Geometry: see drawing. Coordinates: mm, zero at the bounding-box minimum. Give positions to 0.01 mm unless a question says otherwise; leave off trailing zeros. Write each loop counter-clockwise with the first axis right and the second up, starting at its lowest first coordinate (ties: lowest second). Pieces come first, ordered by that corner, then holes. Notation, with made-up numbers: (11, 64.5) -> (21, 64.5) arc R30 cw to (21, 98.5) -> close; hole circle Ø3 at (36, 83). An arc over 180 degrees is marked (long way). Use one line per item in the form item = value. Start each with the question number.
(1) Cut plane C-C, the plane z = 5.5. Output: boundary loops of the cut face in (x, y), and give its area (3 significant figures).
(2) Cut plane B-B, the plane y = 6.5. Output: boundary loops of the cut face in (x, z).
(3) Cut plane D-D, the plane x = 4.25. Output: boundary loops of the cut face in (y, z).
(4) Cut plane A-A, the plane x = 6.5. Output: boundary loops of the cut face in (y, z).
(5) Material intervals for line 1 along Y through (x, z) = (6.5, 2.5); line 2 along X through (y, z) = (6.5, 9.25); line 3 along Y through (x, z) = (7.75, 1.5), sorted ascending. Write a range as from..to.
(6) Draft query along Y for the marked faces 1, 2, 3 and 4. Return one class per face: pulls with the +Y half, pulls with the -Y half, needs draft (parallel to the pull), parting line crosses it, or undercut.
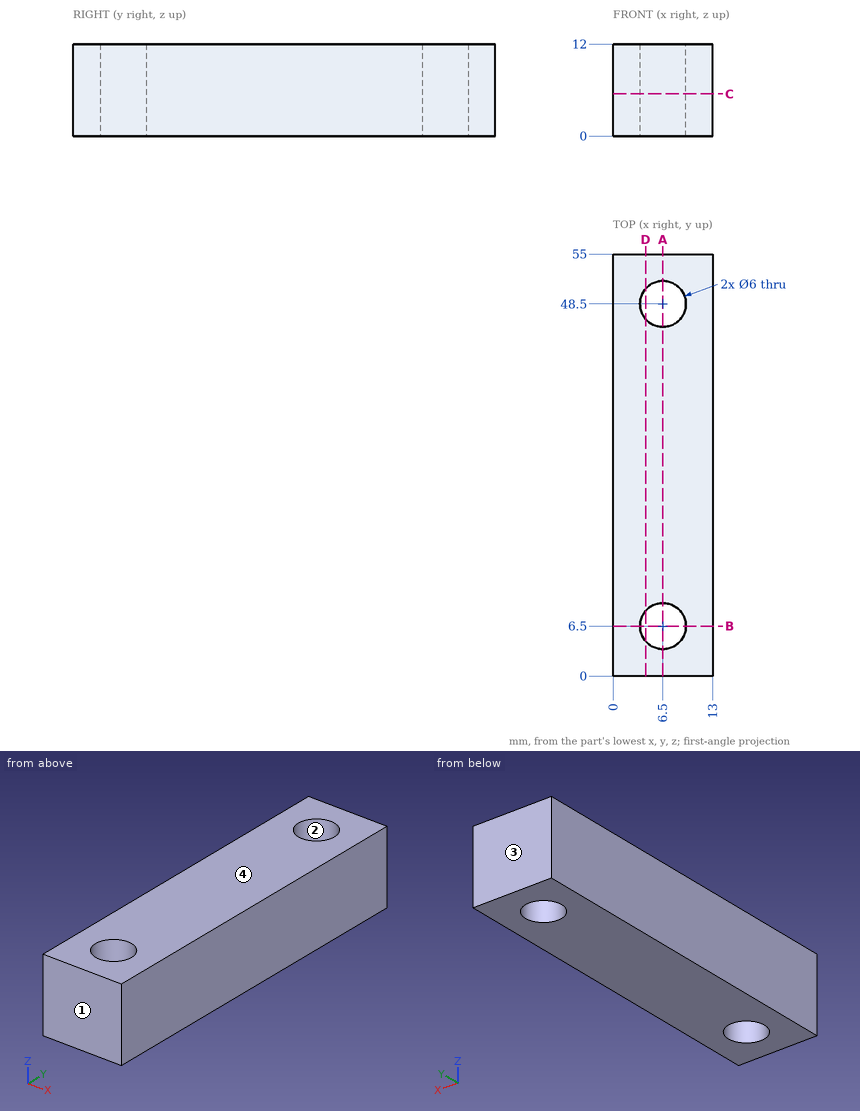
Geometry says:
q1.outline = (0, 0) -> (13, 0) -> (13, 55) -> (0, 55) -> close; hole circle Ø6 at (6.5, 6.5); hole circle Ø6 at (6.5, 48.5)
q1.area = 658 mm^2
q2.outline = (0, 0) -> (3.5, 0) -> (3.5, 12) -> (0, 12) -> close; (9.5, 0) -> (13, 0) -> (13, 12) -> (9.5, 12) -> close
q3.outline = (0, 0) -> (4.52, 0) -> (4.52, 12) -> (0, 12) -> close; (8.48, 0) -> (46.52, 0) -> (46.52, 12) -> (8.48, 12) -> close; (50.48, 0) -> (55, 0) -> (55, 12) -> (50.48, 12) -> close
q4.outline = (0, 0) -> (3.5, 0) -> (3.5, 12) -> (0, 12) -> close; (9.5, 0) -> (45.5, 0) -> (45.5, 12) -> (9.5, 12) -> close; (51.5, 0) -> (55, 0) -> (55, 12) -> (51.5, 12) -> close
q5.line_1 = 0..3.5, 9.5..45.5, 51.5..55
q5.line_2 = 0..3.5, 9.5..13
q5.line_3 = 0..3.77, 9.23..45.77, 51.23..55
q6.face_1 = pulls with the -Y half
q6.face_2 = undercut
q6.face_3 = pulls with the +Y half
q6.face_4 = needs draft
